Build history of the part. All positions in model axes, mm. Face numbers are marked on the shaded views. A direction names the side the tool comes from. Round coordinates to 2 decimals unless told otherwise and drop trailing zeros. Loops run counter-clockwise (first coordinate to the right, second up) from the corner with the lowest first, then second, coordinate; pieces in that order, holes last.
from build123d import *

# Parameters (mm, degrees)
PAD_DEPTH            = 19
FILLET001_R          = 6.35
POCKET002_DEPTH      = 14.001
SKETCH014_R          = 1
POCKET005_DEPTH      = 0.001
POCKET005_DEPTH_BACK = 19.001
SKETCH015_R          = 3
POCKET006_DEPTH      = 3


with BuildPart() as part:
    # Sketch001 → Pad (new body)
    with BuildSketch(Plane.XY):
        with BuildLine():
            Line((180, 175), (180, 31.35))
            ThreePointArc((173.65, 25), (178.140128, 26.859872), (180, 31.35))
            Line((173.65, 25), (124.577301, 25))
            ThreePointArc((124.577301, 25), (121.333458, 24.108936), (119, 21.685821))
            Line((119, 21.685821), (109, 3.314179))
            ThreePointArc((103.422699, 0), (106.666542, 0.891064), (109, 3.314179))
            Line((103.422699, 0), (6.35, 0))
            ThreePointArc((0, 6.35), (1.859872, 1.859872), (6.35, 0))
            Line((0, 98.8), (0, 6.35))
            ThreePointArc((76.2, 175), (22.318463, 152.681537), (0, 98.8))
            Line((180, 175), (76.2, 175))
        make_face()
    extrude(amount=PAD_DEPTH)

    # Fillet001
    fillet001_edges = [part.edges().sort_by_distance(p)[0] for p in [
        (180, 175, 9.5),
    ]]
    fillet(fillet001_edges, radius=FILLET001_R)

    # Sketch007 → Pocket002 (cut, through all)
    with BuildSketch(Plane.XY.offset(5)):
        with BuildLine():
            Line((165, 170), (121, 170))
            Line((121, 170), (71.17245, 141.232051))
            Line((71.17245, 141.232051), (86.028857, 115.5))
            Line((86.028857, 115.5), (125, 138))
            Line((125, 138), (175, 138))
            Line((175, 138), (175, 160))
            ThreePointArc((165, 170), (167.928932, 162.928932), (175, 160))
        make_face()
    extrude(amount=POCKET002_DEPTH, mode=Mode.SUBTRACT)

    # Sketch014 → Pocket005 (cut, two sides)
    with BuildSketch(Plane.XY) as pocket005_sk:
        with Locations((172, 167)):
            Circle(SKETCH014_R)
        with Locations((127, 33)):
            Circle(SKETCH014_R)
    extrude(amount=-POCKET005_DEPTH, mode=Mode.SUBTRACT)
    extrude(pocket005_sk.sketch, amount=POCKET005_DEPTH_BACK, mode=Mode.SUBTRACT)

    # Sketch015 → Pocket006 (cut)
    with BuildSketch(Plane.XY):
        with Locations((127, 33)):
            Circle(SKETCH015_R)
        with Locations((172, 167)):
            Circle(SKETCH015_R)
    extrude(amount=POCKET006_DEPTH, mode=Mode.SUBTRACT)


solid = part.part
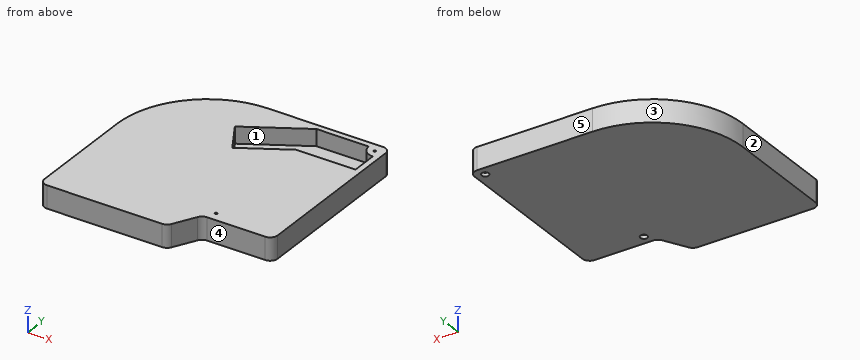
(1) Probe line 1 (Y direction, x = 127, z = 12); line 2 (X direction, y = 33, z = 10); line 3 (Y direction, x = 172, z = 0.85). List the from-to ranges inside material, lowest first.
Responses:
line 1: y = 25 to 32, 34 to 138, 170 to 175
line 2: x = 0 to 126, 128 to 180
line 3: y = 25 to 164, 170 to 175
(2) Slice it at A-A on z = 9. List the corners of the cut face in (x, y), plus the area to 3 significant figures.
Responses:
outline: (0, 6.35) arc R6.35 ccw to (6.35, 0) - (103.42, 0) arc R6.35 ccw to (109, 3.31) - (119, 21.69) arc R6.35 cw to (124.58, 25) - (173.65, 25) arc R6.35 ccw to (180, 31.35) - (180, 168.65) arc R6.35 ccw to (173.65, 175) - (76.2, 175) arc R76.2 ccw to (0, 98.8) - close; hole (71.17, 141.23) - (86.03, 115.5) - (125, 138) - (175, 138) - (175, 160) arc R10 cw to (165, 170) - (121, 170) - close; hole circle Ø2 at (127, 33); hole circle Ø2 at (172, 167)
area: 25,500 mm2
(3) Slice it at C-C on x = 97. List the corners of the cut face in (y, z).
Responses:
outline: (0, 0) - (175, 0) - (175, 19) - (156.14, 19) - (156.14, 5) - (121.83, 5) - (121.83, 19) - (0, 19) - close
(4) Which spindle directions (+Z, -Z, +X, -X, +Y, -Y) get a long thin tool onto all of the face, cutting with end or side? Do the marked faces 4 and 5. Say none if no direction does.
Responses:
face 4: +Z, -Z, +X, -Y
face 5: +Z, -Z, +X, -X, +Y
(5) Slice it at D-D on y = 17. List the corners of the cut face in (x, z).
Responses:
outline: (0, 0) - (116.45, 0) - (116.45, 19) - (0, 19) - close
(6) Slice it at B-B on y = 134. List the corners of the cut face in (x, z).
Responses:
outline: (8.62, 0) - (180, 0) - (180, 19) - (118.07, 19) - (118.07, 5) - (75.35, 5) - (75.35, 19) - (8.62, 19) - close
(7) Pin check, flat tips, straight feed: P1, Ø2.5, axis at x = 127, y = 33, coming from the -Z side; P2, Ø4, axis at x = 152, z = 10, coming from the -Y side; P3, Ø7, axis at y = 148.5, z = 12.5, coming from the -X side. Stop position of each tip, or through.
Responses:
P1: stops at z = 3
P2: stops at y = 25
P3: stops at x = 15.6
(8) Pull direction Y, two halves, no side cores. Call the marked faces 1, 2 and 3: +Y half, -Y half, draft (parallel to the pull), parting line (faces both ways), or undercut.
Responses:
face 1: undercut
face 2: draft
face 3: +Y half
